Could you check a few things on this model? Use its own coordinates, in mm. Face numbers are marked on the shaded views. A direction names the side the tool comes from. Round coordinates to 2 decimals unless told otherwise and drop trailing zeros. Loops run counter-clockwise (first coordinate to the right, second up) from the corner with the lowest first, then second, coordinate; pieces in that order, holes last. Notation, with made-up numbers: M 18,63 L 48,63 A33 cw 48,97 Z; hole C 8.25,71 d7. An arc over 180 degrees is marked long. Answer in a Markdown table with one row per item.
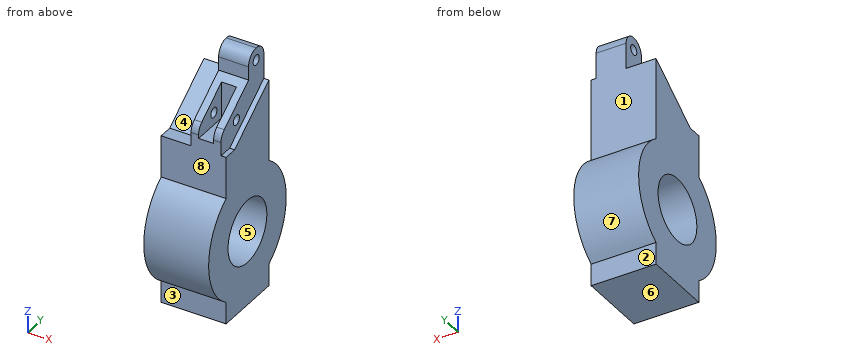
```python
from build123d import *

# Parameters (mm, degrees)
SKETCH1_R           = 1
SKETCH1_R_2         = 6.35
BOSS_EXTRUDE1_DEPTH = 9
SKETCH2_W           = 6
SKETCH2_H           = 6.5
BOSS_EXTRUDE2_DEPTH = 5
CUT_EXTRUDE1_REACH  = 54.627
SKETCH3_R           = 1
FILLET1_R           = 2.5
SKETCH4_W           = 3
SKETCH4_H           = 8
CUT_EXTRUDE3_DEPTH  = 7.5
CUT_EXTRUDE8_DEPTH  = 6
CUT_EXTRUDE9_DEPTH  = 6
SKETCH9_W           = 49.64202669
SKETCH9_H           = 25.4
CUT_EXTRUDE11_DEPTH = 5


with BuildPart() as part:
    # Sketch1 → Boss-Extrude1 (new, symmetric)
    with BuildSketch(Plane(origin=(0, 0, 0), x_dir=(0, 0, -1), z_dir=(1, 0, 0))):
        with BuildLine():
            Line((-45.176360368, 3.046904516), (-38.74778894, -5.953095484))
            ThreePointArc((-38.74778894, -5.953095484), (-37.857409214, -6.722919107), (-36.713455262, -7))
            Line((-36.713455262, -7), (-25.596697599, -7))
            ThreePointArc((-25.596697599, -7), (-15, -12.7), (-4.403302401, -7))
            Line((-4.403302401, -7), (0, -7))
            Line((0, -7), (0, 7))
            Line((0, 7), (-4.403302401, 7))
            ThreePointArc((-4.403302401, 7), (-15, 12.7), (-25.596697599, 7))
            Line((-25.596697599, 7), (-43.14202669, 7))
            ThreePointArc((-43.14202669, 7), (-45.364945797, 5.643953952), (-45.176360368, 3.046904516))
        make_face()
        with Locations((-38.499169547, -2)):
            Circle(SKETCH1_R, mode=Mode.SUBTRACT)
        with Locations((-15, 0)):
            Circle(SKETCH1_R_2, mode=Mode.SUBTRACT)
    extrude(amount=BOSS_EXTRUDE1_DEPTH, both=True)

    # Sketch2 → Boss-Extrude2 (add)
    with BuildSketch(Plane(origin=(0, 7, 0), x_dir=(1, 0, 0), z_dir=(0, 1, 0))):
        with Locations((0, -46.39202669)):
            Rectangle(SKETCH2_W, SKETCH2_H)
    extrude(amount=-BOSS_EXTRUDE2_DEPTH)

    # Sketch3 → Cut-Extrude1 (cut, up to next)
    with BuildSketch(Plane(origin=(3, 0, 0), x_dir=(0, 0, -1), z_dir=(1, 0, 0)), mode=Mode.PRIVATE) as cut_extrude1_sk1:
        with Locations((-47.14202669, 4.5)):
            Circle(SKETCH3_R)
    cut_extrude1_tool1 = extrude(cut_extrude1_sk1.sketch, amount=-CUT_EXTRUDE1_REACH, mode=Mode.PRIVATE) & part.part
    add(cut_extrude1_tool1.solids().sort_by_distance((3, 4.5, 47.142027))[0], mode=Mode.SUBTRACT)

    # Fillet1
    fillet1_edges = [part.edges().sort_by_distance(p)[0] for p in [
        (0, 2, 49.64202669),
        (0, 7, 49.64202669),
    ]]
    fillet(fillet1_edges, radius=FILLET1_R - 0.0001)  # a hair under: the kernel refuses the full size

    # Sketch4 → Cut-Extrude3 (cut)
    with BuildSketch(Plane.XZ.offset(7)):
        with Locations((0, 39.99778894)):
            Rectangle(SKETCH4_W, SKETCH4_H)
    extrude(amount=-CUT_EXTRUDE3_DEPTH, mode=Mode.SUBTRACT)

    # Sketch6 → Cut-Extrude8 (cut)
    with BuildSketch(Plane(origin=(9, 0, 0), x_dir=(0, 0, -1), z_dir=(1, 0, 0))):
        Polygon((-48, 7), (-38, -7), (-34, -7), (-34, -4.2), (-42, 7), align=None)
    extrude(amount=-CUT_EXTRUDE8_DEPTH, mode=Mode.SUBTRACT)

    # Sketch8 → Cut-Extrude9 (cut)
    with BuildSketch(Plane.ZY.offset(9)):
        Polygon((38, -7), (48, 7), (42, 7), (34, -4.2), (34, -7), align=None)
    extrude(amount=-CUT_EXTRUDE9_DEPTH, mode=Mode.SUBTRACT)

    # Sketch9 → Cut-Extrude11 (cut)
    with BuildSketch(Plane(origin=(9, 0, 0), x_dir=(0, 0, -1), z_dir=(1, 0, 0))):
        with Locations((-24.821013345, 0)):
            Rectangle(SKETCH9_W, SKETCH9_H)
    extrude(amount=-CUT_EXTRUDE11_DEPTH, mode=Mode.SUBTRACT)


solid = part.part
```
1) Will these pins go through, and if not, where does the flat tip stop? P1, Ø0.8, axis at x = -1, z = 46.5, coming from the -Y side; P2, Ø5, axis at x = -1.5, y = 8.5, coming from the +Z side; P3, Ø2.5, axis at y = -2, z = 38.5, coming from the +X side.
Computed:
| item | result |
|---|---|
| P1 | stops at y = 2 |
| P2 | stops at z = 49.14 |
| P3 | stops at x = 3 |
2) I want a section at D-D, the plane x = 0.75. State how many separate pieces and enclosed holes the cut face has, plus the area to 3 significant figures.
Computed:
| item | result |
|---|---|
| separate pieces | 1 |
| enclosed holes | 2 |
| area | 622 mm² |
3) I want a section at C-C, the plane x = -5. Please give me the cut outline in (y, z), plus the area to 3 significant figures.
Computed:
| item | result |
|---|---|
| outline | M -7,0 L 7,0 L 7,4.4 A12.7 ccw 7,25.6 L 7,42 L -4.2,34 L -7,34 L -7,25.6 A12.7 ccw -7,4.4 Z; hole C 0,15 d12.7 |
| area | 564 mm² |
4) I want a section at B-B, the plane z = 15. Please give me the cut outline in (x, y), plus the area to 3 significant figures.
Computed:
| item | result |
|---|---|
| outline | M -9,-12.7 L 4,-12.7 L 4,-6.35 L -9,-6.35 Z; M -9,6.35 L 4,6.35 L 4,12.7 L -9,12.7 Z |
| area | 165 mm² |
5) I want a section at A-A, the plane y = 0. Please give me the cut outline in (x, z).
Computed:
| item | result |
|---|---|
| outline | M -9,0 L 4,0 L 4,8.65 L -9,8.65 Z; M -9,21.35 L 4,21.35 L 4,37 L 3,37 L 3,43 L 1.5,43 L 1.5,36 L -1.5,36 L -1.5,43 L -3,43 L -3,37 L -9,37 Z |
6) If we mould it in two halves opening along Y, with no side actions, what happens to the marked faces 5, 6, 7 and 8? For each: released by +Y, released by -Y, zero draft, split by the parting line, or undercut.
Computed:
| item | result |
|---|---|
| face 5 | undercut |
| face 6 | zero draft |
| face 7 | released by +Y |
| face 8 | released by -Y |
7) I need wall thicknesses on line 1 (X direction, y = -2.5, z = 41); line 2 (Y direction, x = -5.5, z = 15); line 3 (Z direction, x = -2.05, y = -2). Which ranges of each line are inside material? Lowest first, please.
Computed:
| item | result |
|---|---|
| line 1 | x = -3 to -1.5, 1.5 to 3 |
| line 2 | y = -12.7 to -6.35, 6.35 to 12.7 |
| line 3 | z = 0 to 8.97, 21.03 to 37.5, 39.5 to 41.57 |
8) Which directions (+Z, -Z, +X, -X, +Y, -Y) give clear straight access to the entire face, cutting with the end or side of a thin tool? Please do the marked faces 1, 2, 3 and 4.
Computed:
| item | result |
|---|---|
| face 1 | +Z, +X, -X, +Y |
| face 2 | -Z, +X, -X, +Y |
| face 3 | -Z, +X, -X, -Y |
| face 4 | +Z, -X, -Y |
